Input: part model. Units: mm. Frame: model coordinates. A direction names the side the tool comes from. Give positions to 0.01 mm unless a question says otherwise; leave off trailing zeros. Loops run counter-clockwise (first coordinate to the right, second up) from the corner with the lowest first, then second, coordinate; pieces in that order, holes last. Notation, with made-up numbers: M 54,-7 L 97,-7 A33 cw 97,21 Z; hole C 68,4 d5. An arc over 180 degrees is marked long. Answer as a JSON object with one key per item and string values. Group by question number.
1) First-contact query: P1, Ø8, axis at y = 26, z = 5, coming from the +X side; P2, Ø10, axis at x = 7, z = 5.5, coming from the +Y side; P3, Ø10, axis at y = -30.5, z = 1, coming from the -X side; P4, Ø4, axis at y = 33, z = 3, coming from the +X side. Flat tips, straight axial feed; report the tip coordinate or a pass-through.
2) Section query C-C on z = -3. Return loops of the section in (x, y).
3) Section query D-D on z = 7.5. Return loops of the section in (x, y).
4) Draft query along X for faces 3 (the flat face through (0, -7, -6)), 4 (the conical face through (5.26, -23.67, 8.75)), 5 (the flat face through (-9, 1, -10)). Return one class per face: +X half, -X half, draft (parallel to the pull), parting line (faces both ways), or undercut.
5) Ray query, L1, parallel to Z at x = -8, y = 10; L2, parallel to X at y = -23, z = -4.25; L3, parallel to Y at x = -27, z = -2.5. Return the intervals inside material, ascending.
6) Access query for faces 1 (the flat face through (0, -5, 10)), 2 (the cylindrical face through (0.867, -3.905, -0.084)). Directions: +Z, -Z, +X, -X, +Y, -Y. A direction counts if a zero-diameter tool reaches every point of the face in a straight line with its end or side. Return the directions, or none.
7) Section query A-A on x = 0. Return loops of the section in (y, z).
from build123d import *

# Parameters (mm, degrees)
F3_D = 3.3


with BuildPart() as f1:
    # F0 (on Front) → F1 (revolve)
    with BuildSketch(Plane.XZ):
        Polygon((0, 10), (-23, 10), (-43, -10), (0, -10), align=None)
        Polygon((-33.3431457505, -6), (-21.3431457505, 6), (-4, 6), (-4, -6), align=None, mode=Mode.SUBTRACT)
    revolve(axis=Axis((0, 0, 0), (0, 0, -1)))

    # F3 (through all)
    with Locations(Plane.XY.offset(10)):
        with Locations((0, 0)):
            Hole(F3_D / 2)


solid = f1.part
Output:
{
 "1": {"P1": "stops at x = 20.41", "P2": "stops at y = 31.84", "P3": "stops at x = -23.23", "P4": "passes through"},
 "2": {"outline": "C 0,0 d72; C 0,0 d8; hole C 0,0 d60.69; hole C 0,0 d3.3"},
 "3": {"outline": "C 0,0 d51; hole C 0,0 d3.3"},
 "4": {"face 3": "undercut", "face 4": "parting line", "face 5": "draft"},
 "5": {"L1": "z = -10 to -6, 6 to 10", "L2": "x = -29.3 to -21.66, 21.66 to 29.3", "L3": "y = -23.05 to -12.71, 12.71 to 23.05"},
 "6": {"face 1": "+Z, +X, -X, +Y, -Y", "face 2": "none"},
 "7": {"outline": "M -43,-10 L -1.65,-10 L -1.65,10 L -23,10 Z; M 1.65,-10 L 43,-10 L 23,10 L 1.65,10 Z; hole M -33.34,-6 L -4,-6 L -4,6 L -21.34,6 Z; hole M 4,-6 L 33.34,-6 L 21.34,6 L 4,6 Z"}
}
